```python
from build123d import *

# Parameters (mm, degrees)
F1_DEPTH = 500
F2_W     = 400
F2_H     = 400
F3_DEPTH = 150
F4_R     = 100
F4_R_2   = 50
F5_DEPTH = 25
F6_DEPTH = 200


with BuildPart() as f1:
    # F0 (on Front) → F1 (new body)
    with BuildSketch(Plane.XZ):
        Polygon((-1000, 0), (0, 0), (0, 100), (-250, 100), (-250, 350), (-750, 350), (-750, 100), (-1000, 100), align=None)
    extrude(amount=F1_DEPTH)

    # F2 (on face) → F3 (cut)
    with BuildSketch(Plane.XY.offset(350)):
        with Locations((-500, -250)):
            Rectangle(F2_W, F2_H)
    extrude(amount=-F3_DEPTH, mode=Mode.SUBTRACT)

    # F4 (on face) → F5 (cut)
    with BuildSketch(Plane.XY.offset(200)):
        with Locations((-500, -250)):
            Circle(F4_R)
        with Locations((-500, -250)):
            Circle(F4_R_2, mode=Mode.SUBTRACT)
    extrude(amount=-F5_DEPTH, mode=Mode.SUBTRACT)

    # F4 (on face) → F6 (cut)
    with BuildSketch(Plane.XY.offset(200)):
        with Locations((-500, -250)):
            Circle(F4_R_2)
    extrude(amount=-F6_DEPTH, mode=Mode.SUBTRACT)


solid = f1.part
```
The listing builds one solid part. Answer for the finished solid, in the listing's coordinates (mm). A direction names the side the tool comes from. Round coordinates to 2 decimals unless told otherwise and drop trailing zeros. Order: outer loops, then holes, each group sorted by start corner. A loop starts at its lowest first (then second) coordinate and runs counter-clockwise, first axis right, second up. Notation, with made-up numbers: (25, 78.5) - (42, 78.5) arc R26 cw to (42, 99.5) - close; hole circle Ø8 at (-22.75, -32). An arc over 180 degrees is marked (long way). Put each result on its own line as item: value. Start each with the question number.
(1) Find section D-D (z = 252.5). Give the vertices of the cut face in (x, y).
(2) Straight lines are drawn through the part: probe 1 along X at (y, z) = (-196, 289); probe 2 along Y at (x, z) = (-500, 191.75); probe 3 along Y at (x, z) = (-567.5, 231.5). For each, find the intervals that lie inside material, in ascending order. Write a range as from..to.
(3) Determine the mould class of faces 1 (the flat face through (-507, 0, 139)), 2 (the flat face through (-592, -203, 200)), 3 (the cylindrical face through (-599.903, -245.603, 187.675)), 4 (the flat face through (-719, -246, 350)) for opening direction Y: released by +Y, released by -Y, zero draft, split by the parting line, or undercut.
(4) Find section A-A (y = -250). Give the vertices of the cut face in (x, z).
(5) Given P1, Ø1.5, axis at y = -310.5, z = 116.5, coming from the +X side; P2, Ø12, axis at y = -65.5, z = 178.5, coming from the -X side, each flat-ended and moving along its own axis, determine where each tip first touches the part or whether it passes through.
(6) Find section B-B (x = -500). Give the vertices of the cut face in (y, z), plus the area to 3 significant figures.
(7) Find section C-C (z = 80.5). Give the vertices of the cut face in (x, y).
(8) For faces 5 (the flat face through (-123, -246, 100)), 6 (the flat face through (-873, -246, 100)), 7 (the cylindrical face through (-452.31, -234.98, 88.72)), 8 (the flat face through (-300, -253, 276)), determine the directions among +Z, -Z, +X, -X, +Y, -Y from which every point of the face is accessible in a straight line to the end or side of a thin tool.
Reply:
1. outline: (-750, -500) - (-250, -500) - (-250, 0) - (-750, 0) - close; hole (-700, -450) - (-300, -450) - (-300, -50) - (-700, -50) - close
2. probe 1: -750..-700, -300..-250
2. probe 2: -500..-350, -150..0
2. probe 3: -500..-450, -50..0
3. face 1: released by +Y
3. face 2: undercut
3. face 3: undercut
3. face 4: zero draft
4. outline: (-1000, 0) - (-550, 0) - (-550, 175) - (-600, 175) - (-600, 200) - (-700, 200) - (-700, 350) - (-750, 350) - (-750, 100) - (-1000, 100) - close; (-450, 0) - (0, 0) - (0, 100) - (-250, 100) - (-250, 350) - (-300, 350) - (-300, 200) - (-400, 200) - (-400, 175) - (-450, 175) - close
5. P1: x = -250
5. P2: x = -750
6. outline: (-500, 0) - (-300, 0) - (-300, 175) - (-350, 175) - (-350, 200) - (-450, 200) - (-450, 350) - (-500, 350) - close; (-200, 0) - (0, 0) - (0, 350) - (-50, 350) - (-50, 200) - (-150, 200) - (-150, 175) - (-200, 175) - close
6. area: 92,500 mm^2
7. outline: (-1000, -500) - (0, -500) - (0, 0) - (-1000, 0) - close; hole circle Ø100 at (-500, -250)
8. face 5: +Z, +X, +Y, -Y
8. face 6: +Z, -X, +Y, -Y
8. face 7: +Z, -Z
8. face 8: +Z
